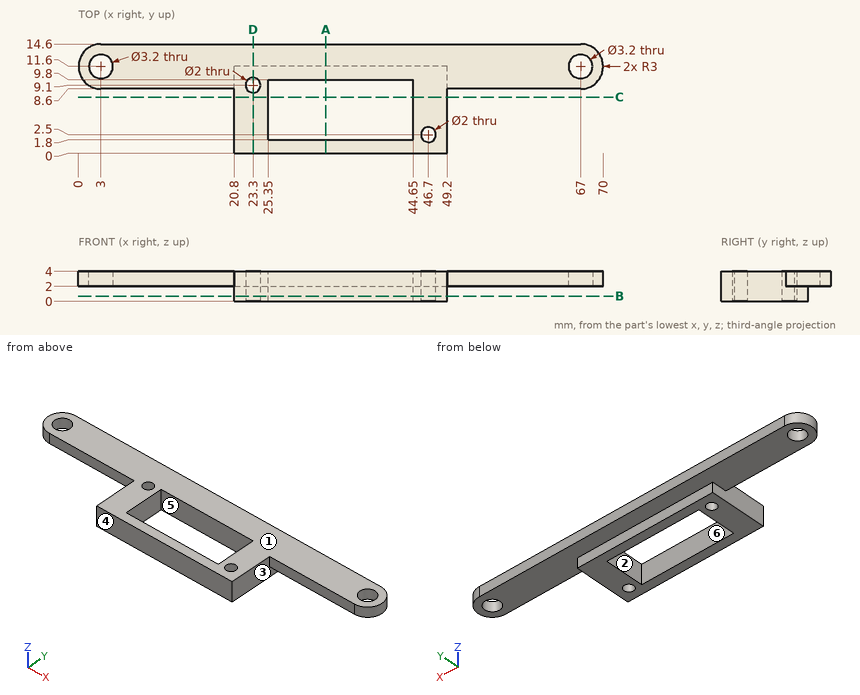
Design review of the part shown in the three views and the two pictorial views. Dimensions are in mm from the part's minimum x, y and z. A direction names the side the tool comes from. Round coordinates to 2 decimals unless told otherwise and drop trailing zeros. Write each loop counter-clockwise with the first axis right and the second up, starting at its lowest first coordinate (ties: lowest second). Pieces come first, ordered by that corner, then holes. Notation, with made-up numbers: M 78,1 L 131,1 A14 ccw 131,21 Z; hole C -34.75,65 d8. An arc over 180 degrees is marked long. One line per item, written item: value. Start each with the question number.
1. Clearance check with flat-ended pins moving along their axes: P1, Ø8, axis at x = 56, y = 4.5, coming from the +Z side; P2, Ø1.6, axis at x = 58.5, z = 2.5, coming from the -Y side; P3, Ø1.2, axis at y = 7, z = 1.5, coming from the -X side; P4, Ø1.5, axis at y = 5, z = 3.5, coming from the +X side. State where each tip first meets the part, or that it passes through.
2. Take a section at A-A on x = 33. State the section outline as (y, z) points, then the cut area to 3 significant figures.
3. For the marked faces 1 and 2, list the 3-axis set-ups (+Z, -Z, +X, -X, +Y, -Y) from which the entire face can be reached by the end or side of a thin tool; tool diameter is ignored.
4. Take a section at C-C on y = 7.5. State the section outline as (x, z) points.
5. Take a section at B-B on z = 0.7. State the section outline as (x, y) points, then the cut area to 3 significant figures.
6. To check wall thickness, follow probe 1 along Y at (x, z) = (46.7, 3.05); probe 2 along Y at (x, z) = (67, 3); probe 3 along X at (y, z) = (8.25, 1.25). State the ranges of each line that lie inside material, in increasing order. Write a range as from..to.
7. Take a section at D-D on x = 23.3. State the section outline as (y, z) points.
8. Draft analysis for pull direction Y (two halves, no side actions). For the marked faces 3, 4, 5 and 6, state which applies: pulls with the +Y half, pulls with the -Y half, needs draft (parallel to the pull), parting line crosses it, or undercut.
Computed:
1. P1: passes through
1. P2: stops at y = 8.6
1. P3: stops at x = 20.8
1. P4: stops at x = 49.2
2. outline: M 0,0 L 1.8,0 L 1.8,4 L 0,4 Z; M 9.8,0 L 11.6,0 L 11.6,2 L 14.6,2 L 14.6,4 L 9.8,4 Z
2. area: 20.4 mm²
3. face 1: +Z, +X, -X, +Y, -Y
3. face 2: +Z, -Z
4. outline: M 20.8,0 L 25.35,0 L 25.35,4 L 20.8,4 Z; M 44.65,0 L 49.2,0 L 49.2,4 L 44.65,4 Z
5. outline: M 20.8,0 L 49.2,0 L 49.2,11.6 L 20.8,11.6 Z; hole C 23.3,9.1 d2; hole M 25.35,1.8 L 44.65,1.8 L 44.65,9.8 L 25.35,9.8 Z; hole C 46.7,2.5 d2
5. area: 169 mm²
6. probe 1: y = 0..1.5, 3.5..14.6
6. probe 2: y = 8.6..10, 13.2..14.6
6. probe 3: x = 20.8..22.77, 23.83..25.35, 44.65..49.2
7. outline: M 0,0 L 8.1,0 L 8.1,4 L 0,4 Z; M 10.1,0 L 11.6,0 L 11.6,2 L 14.6,2 L 14.6,4 L 10.1,4 Z
8. face 3: needs draft
8. face 4: pulls with the -Y half
8. face 5: undercut
8. face 6: undercut
